Geometry check sheet. Reference: the model listing, model coordinates, mm. A direction names the side the tool comes from. Coordinates: 2 decimals unless noted, no trailing zeros. Loops run counter-clockwise (first coordinate to the right, second up) from the corner with the lowest first, then second, coordinate; pieces in that order, holes last.
from build123d import *

# Parameters (mm, degrees)
Y_KSEKLIK_EKSTR_ZYON1_DEPTH = 10
CUT_EXTRUDE1_DEPTH          = 10


with BuildPart() as part:
    # Çizim1 → Yükseklik-Ekstrüzyon1 (new body)
    with BuildSketch(Plane.XY):
        Polygon((-210, 28), (-210, 0), (0, 0), (0, 28), (-15.3, 70), (-60, 70), (-60, 210), (-88, 210), align=None)
    extrude(amount=Y_KSEKLIK_EKSTR_ZYON1_DEPTH)

    # Sketch1 → Cut-Extrude1 (cut)
    with BuildSketch(Plane(origin=(0, 0, 0), x_dir=(-1, 0, 0), z_dir=(0, 0, -1))):
        Polygon((152, 150.469052626), (245.176581689, 150.469052626), (245.176581689, -14.338775046), (152, -14.338775046), (152, 50.347137768), (88, 210), (152, 210), align=None)
    extrude(amount=-CUT_EXTRUDE1_DEPTH, mode=Mode.SUBTRACT)


solid = part.part
1) Section check C-C on y = 40. Record the cut outline in (x, z).
Data:
outline: (-152, 0) - (-4.37, 0) - (-4.37, 10) - (-152, 10) - close
2) Depth check by flat-ended pin: pin 1 (5 mm diameter, centred on x = -41, z = 3, fed in from +Y); pin 2 (1 mm diameter, centred on x = -134.5, z = 2.5, fed in from +Y); pin 3 (5 mm diameter, centred on y = 107.5, z = 4, fed in from +X). Enter the tip coordinate at first touch or a pass-through.
Data:
pin 1: stops at y = 70
pin 2: stops at y = 95.25
pin 3: stops at x = -60
3) Section check A-A on z = 6. Record the cut outline in (x, y).
Data:
outline: (-152, 0) - (0, 0) - (0, 28) - (-15.3, 70) - (-60, 70) - (-60, 210) - (-88, 210) - (-152, 50.35) - close
4) Access from +Z, -Z, +X, -X, +Y, -Y to the whole of each face (thin tool, end or side, straight path). Record for faces 1 (the flat face through (-60, 139, 5)), 2 (the flat face through (-77, 83, 10)).
Data:
face 1: +Z, -Z, +X, +Y
face 2: +Z, +X, -X, +Y, -Y
5) Material ranges on probe 1 along Y at (x, z) = (-40, 2.5); probe 2 along X at (y, z) = (160, 4); probe 3 along X at (y, z) = (75.5, 6.75), recorded low to high.
Data:
probe 1: y = 0 to 70
probe 2: x = -108.04 to -60
probe 3: x = -141.92 to -60
6) Section check B-B on x = -50.5. Record the cut outline in (y, z), and give its area (3 significant figures).
Data:
outline: (0, 0) - (70, 0) - (70, 10) - (0, 10) - close
area: 700 mm2
